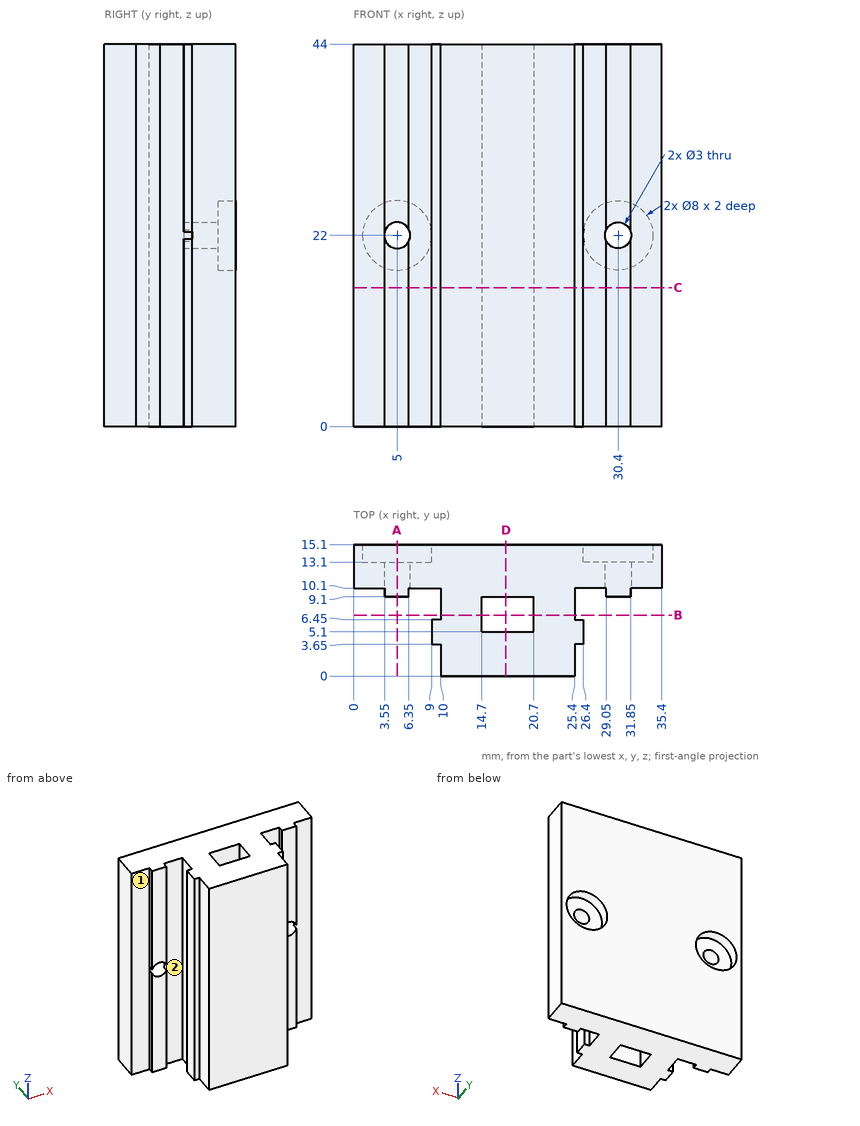
Here's the drawing with two shaded views (mm, measured from the low corner). I have some questions. Give positions to 0.01 mm unless a question says otherwise; leave off trailing zeros. Order: outer loops, then holes, each group sorted by start corner. A loop starts at its lowest first (then second) coordinate and runs counter-clockwise, first axis right, second up. Notation, with made-up numbers: (-26, 48.25) -> (8, 48.25) arc R20 cw to (8, 58.25) -> close; hole circle Ø6 at (17.5, 45.25). An arc over 180 degrees is marked (long way). Use a Markdown table: item, result. Add a question column.
Item 1: Imagine slicing it at A-A on x = 5. Please give me the cut outline in (y, z).
Item 2: Imagine slicing it at B-B on y = 7. Please give me the cut outline in (x, z).
Item 3: Will these pins go through, and if not, where does the flat tip stop? pin 1 (3 mm diameter, centred on x = 30, z = 12.5, fed in from -Y); pin 2 (1.1 mm diameter, centred on x = 26, z = 14.5, fed in from -Y); pin 3 (0.8 mm diameter, centred on y = 4.5, z = 13.5, fed in from -X).
Item 4: Imagine slicing it at C-C on z = 16. Please give me the cut outline in (x, y).
Item 5: I need wall thicknesses on line 1 (X direction, y = 14.3, z = 22); line 2 (X direction, y = 11.1, z = 22); line 3 (Z direction, x = 30.4, y = 14). Which ranges of each line are inside material? Lowest first, please.
Item 6: Imagine slicing it at D-D on x = 17.5. Please give me the cut outline in (y, z).
Item 7: If we mould it in two halves opening along X, with no side actions, what happens to the marked faces 1 and 2? For each: pulls with the +X half, pulls with the -X half, needs draft (parallel to the pull), parting line crosses it, or undercut.
Data:
| question | item | result |
|---|---|---|
| 1 | outline | (9.1, 0) -> (15.1, 0) -> (15.1, 18) -> (13.1, 18) -> (13.1, 20.5) -> (9.1, 20.5) -> close; (9.1, 23.5) -> (13.1, 23.5) -> (13.1, 26) -> (15.1, 26) -> (15.1, 44) -> (9.1, 44) -> close |
| 2 | outline | (10, 0) -> (14.7, 0) -> (14.7, 44) -> (10, 44) -> close; (20.7, 0) -> (25.4, 0) -> (25.4, 44) -> (20.7, 44) -> close |
| 3 | pin 1 | stops at y = 9.1 |
| 3 | pin 2 | stops at y = 3.65 |
| 3 | pin 3 | stops at x = 9 |
| 4 | outline | (0, 10.1) -> (3.55, 10.1) -> (3.55, 9.1) -> (6.35, 9.1) -> (6.35, 10.1) -> (10, 10.1) -> (10, 6.45) -> (9, 6.45) -> (9, 3.65) -> (10, 3.65) -> (10, 0) -> (25.4, 0) -> (25.4, 3.65) -> (26.4, 3.65) -> (26.4, 6.45) -> (25.4, 6.45) -> (25.4, 10.1) -> (29.05, 10.1) -> (29.05, 9.1) -> (31.85, 9.1) -> (31.85, 10.1) -> (35.4, 10.1) -> (35.4, 15.1) -> (0, 15.1) -> close; hole (14.7, 5.1) -> (20.7, 5.1) -> (20.7, 9.1) -> (14.7, 9.1) -> close |
| 5 | line 1 | x = 0 to 1, 9 to 26.4, 34.4 to 35.4 |
| 5 | line 2 | x = 0 to 3.5, 6.5 to 28.9, 31.9 to 35.4 |
| 5 | line 3 | z = 0 to 18, 26 to 44 |
| 6 | outline | (0, 0) -> (5.1, 0) -> (5.1, 44) -> (0, 44) -> close; (9.1, 0) -> (15.1, 0) -> (15.1, 44) -> (9.1, 44) -> close |
| 7 | face 1 | needs draft |
| 7 | face 2 | undercut |
